Verification items for the finished model (mm, model axes). Coordinates: 2 decimals unless noted, no trailing zeros. Loops run counter-clockwise (first coordinate to the right, second up) from the corner with the lowest first, then second, coordinate; pieces in that order, holes last. Notation, with made-up numbers: (35, 74.25) - (78, 74.25) arc R5 cw to (78, 79.25) - close; hole circle Ø1 at (16.25, 83.25). An arc over 180 degrees is marked (long way). Answer as CSV lines item,"result". Start each with the question number.
1. Cross-section at A-A (x = 4148.5). Enter the section's corners in (y, z), plus the area to 3 significant figures.
2. Material ranges on line 1 (X direction, y = -3184.5, z = 5.9); line 2 (X direction, y = -3140.5, z = 6.05) (3 decimals); line 3 (Y direction, x = 4174.5, z = 5.1), recorded low to high. Write a range as [from, to].
3. Cross-section at B-B (z = 5). State how many separate pieces and enclosed holes the cut face has, plus the area to 3 significant figures.
```python
from build123d import *

# Parameters (mm, degrees)
SKETCH1_R           = 4.000005254
SKETCH1_R_2         = 6.295294196
SKETCH1_R_3         = 6.298818985
SKETCH1_R_4         = 4.000046515
SKETCH1_R_5         = 3.96227159
SKETCH1_R_6         = 6.298583834
SKETCH1_R_7         = 6.289262296
SKETCH1_R_8         = 4.000026217
BOSS_EXTRUDE1_DEPTH = 10
SCALE1_SCALE        = 0.254310345


with BuildPart() as part:
    # Sketch1 → Boss-Extrude1 (new body)
    with BuildSketch(Plane.XY):
        Polygon((4033.100097656, -3054.507080078), (4035.240234375, -3052.350097656), (4259.751464844, -3052.350097656), (4265.899902344, -3058.498535156), (4265.899902344, -3266.751464844), (4249.751464844, -3282.899902344), (4046.248535156, -3282.899902344), (4033.100097656, -3269.751464844), align=None)
        with Locations((4046.000008659, -3063.7500542)):
            Circle(SKETCH1_R, mode=Mode.SUBTRACT)
        with Locations((4143.496433826, -3063.770149106)):
            Circle(SKETCH1_R_2, mode=Mode.SUBTRACT)
        with Locations((4223.5, -3063.750049197)):
            Circle(SKETCH1_R_3, mode=Mode.SUBTRACT)
        with Locations((4252.000063875, -3064.25000712)):
            Circle(SKETCH1_R_4, mode=Mode.SUBTRACT)
        with Locations((4251.021334492, -3237.795441039)):
            Circle(SKETCH1_R_5, mode=Mode.SUBTRACT)
        with Locations((4223.5, -3233.750415039)):
            Circle(SKETCH1_R_6, mode=Mode.SUBTRACT)
        with Locations((4143.493016467, -3233.75871347)):
            Circle(SKETCH1_R_7, mode=Mode.SUBTRACT)
        with Locations((4045.500040954, -3237.749996915)):
            Circle(SKETCH1_R_8, mode=Mode.SUBTRACT)
    extrude(amount=BOSS_EXTRUDE1_DEPTH)


with BuildPart() as part_1:
    # Scale1: scaled about (4149.056874209, -3167.460792727, 5)
    add(part.part.scale(SCALE1_SCALE).moved(Location((3093.90878982, -2361.942746301, 3.728448276))))


solid = part_1.part
```
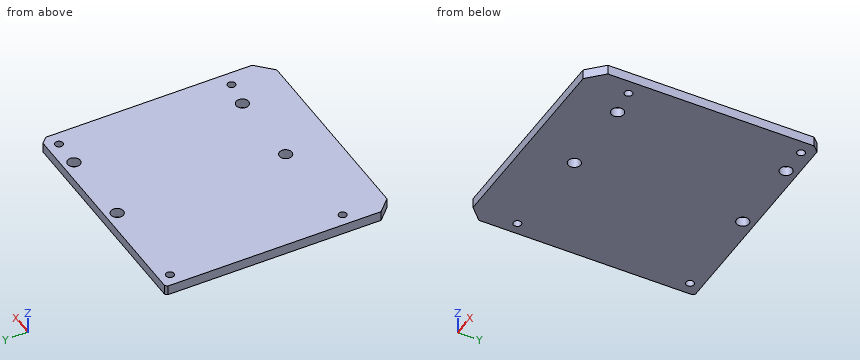
Values follow:
1,outline,"(-3196.82, 3.73) - (-3185.67, 3.73) - (-3185.67, 6.27) - (-3196.82, 6.27) - close; (-3182.97, 3.73) - (-3142.44, 3.73) - (-3142.44, 6.27) - (-3182.97, 6.27) - close; (-3139.74, 3.73) - (-3138.19, 3.73) - (-3138.19, 6.27) - (-3139.74, 6.27) - close"
1,area,"135 mm²"
2,line 1,"x = [4119.57, 4122.14], [4123.3, 4146.05], [4149.23, 4166.4], [4169.58, 4174.44], [4175.53, 4178.77]"
2,line 2,"x = [4119.568, 4122.017], [4123.68, 4146.155], [4149.131, 4166.498], [4169.479, 4174.511], [4175.962, 4178.771]"
2,line 3,"y = [-3196.82, -3186.23], [-3184.47, -3141.92], [-3140.51, -3138.19]"
3,separate pieces,"1"
3,enclosed holes,"8"
3,area,"3,410 mm²"
